```python
from build123d import *

# Parameters (mm, degrees)
F0_W        = 20
F0_H        = 200
F1_DEPTH    = 20
F2_W        = 15
F2_H        = 100
F3_DEPTH    = 20
F6_R        = 7
F7_DEPTH    = 20.001
F8_T1_DEPTH = 20
F9_R        = 20
F11_D       = 6.7564
F11_DEPTH   = 50
F11_TIP     = 2.0298273432


# Not quite as in the source:
# - a fillet or chamfer that OpenCascade refuses, or shapes differently, is made with other operations: its cross-section is extruded or revolved along the edge and cut away or added


with BuildPart() as f1:
    # F0 (on Front) → F1 (new body)
    with BuildSketch(Plane.XZ):
        with Locations((10, 100)):
            Rectangle(F0_W, F0_H)
    extrude(amount=F1_DEPTH)

    # F2 (on face) → F3 (cut)
    with BuildSketch(Plane.YZ.offset(20)):
        with Locations((-12.5, 50)):
            Rectangle(F2_W, F2_H)
    extrude(amount=-F3_DEPTH, mode=Mode.SUBTRACT)

    # F5: sweep along a path in F5_path
    with BuildLine(Plane(origin=(0, -5, 0), x_dir=(0, -1, 0), z_dir=(0, 0, -1))) as f5_path:
        Line((0, 0), (-5, 0))
    # F4 (on face) → F5 (sweep, cut)
    with BuildSketch(Plane(origin=(0, 0, 0), x_dir=(-1, 0, 0), z_dir=(0, 1, 0))):
        with BuildLine():
            Line((0, 0), (0, 10))
            ThreePointArc((0, 10), (-2.9289321881, 2.9289321881), (-10, 0))
            Line((-10, 0), (0, 0))
        make_face()
        with BuildLine():
            ThreePointArc((-10, 0), (-17.0710678277, 2.9289322039), (-20, 10.0000000447))
            Line((-20, 10.0000000447), (-20, 0))
            Line((-20, 0), (-10, 0))
        make_face()
    sweep(path=f5_path.line, mode=Mode.SUBTRACT)

    # F6 (on face) → F7 (cut, through all)
    with BuildSketch(Plane(origin=(0, 0, 0), x_dir=(-1, 0, 0), z_dir=(0, 1, 0))):
        with Locations((-10, 10)):
            Circle(F6_R)
    extrude(amount=-F7_DEPTH, mode=Mode.SUBTRACT)

    # F8: fillet of radius 45 on 1 edges, made by hand

    # F8_s2 → F8_t1 (join)
    with BuildSketch(Plane.YZ):
        with BuildLine():
            ThreePointArc((-5, 66.4589803375), (-8.9208081871, 84.8301534084), (-20, 100))
            Line((-20, 100), (-5, 100))
            Line((-5, 100), (-5, 66.4589803375))
        make_face()
    extrude(amount=F8_T1_DEPTH)

    # F9
    f9_edges = [f1.edges().sort_by_distance(p)[0] for p in [
        (10, -20, 100),
    ]]
    fillet(f9_edges, radius=F9_R)

    # F11
    with Locations(Plane.XY.offset(200)):
        with Locations((10, -10)):
            Hole(F11_D / 2, depth=F11_DEPTH)
            with Locations((0, 0, -(F11_DEPTH + F11_TIP / 2))):  # 118° drill point
                Cone(0, F11_D / 2, F11_TIP, mode=Mode.SUBTRACT)


solid = f1.part
```
Geometry check sheet. Reference: the model listing, model coordinates, mm. A direction names the side the tool comes from. Give positions to 0.01 mm unless a question says otherwise; leave off trailing zeros. Loops run counter-clockwise (first coordinate to the right, second up) from the corner with the lowest first, then second, coordinate; pieces in that order, holes last. Notation, with made-up numbers: M 44.25,19.5 L 52.25,19.5 A28 ccw 52.25,55.5 Z; hole C 59.5,72.5 d3. An arc over 180 degrees is marked long. Answer as CSV lines item,"result".
Item 1: Cross-section at B-B on z = 61.5. Record the cut outline in (x, y), and give its area (3 significant figures).
Values:
outline,"M 0,-5 L 20,-5 L 20,0 L 0,0 Z"
area,"100 mm²"
Item 2: Access from +Z, -Z, +X, -X, +Y, -Y to the whole of each face (thin tool, end or side, straight path). Record for faces 4 (the flat face through (10, 0, 101)), 5 (the flat face through (10, -5, 33)).
Values:
face 4,"+Z, -Z, +X, -X, +Y"
face 5,"-Z, +X, -X, -Y"
Item 3: Material ranges on line 1 (Z direction, x = 10, y = -3.65); line 2 (Y direction, x = 10, z = 184); line 3 (X direction, y = -10, z = 181.5), recorded low to high.
Values:
line 1,"z = 0 to 3, 17 to 200"
line 2,"y = -20 to -13.38, -6.62 to 0"
line 3,"x = 0 to 6.62, 13.38 to 20"
Item 4: Release check for a two-part mould opening along Y. For faces 1 (the cylindrical face through (10.44, -6.65, 174.65)), 2 (the cylindrical face through (9.86, -7.602, 81.539)), 3 (the flat face through (20, -8, 127)) record: pulls with the +Y half, pulls with the -Y half, needs draft (parallel to the pull), parting line crosses it, or undercut.
Values:
face 1,"undercut"
face 2,"pulls with the -Y half"
face 3,"needs draft"
Item 5: Cross-section at A-A on z = 12.5. Record the cut outline in (x, y), and give its area (3 significant figures).
Values:
outline,"M 0,-5 L 3.46,-5 L 3.46,0 L 0,0 Z; M 16.54,-5 L 20,-5 L 20,0 L 16.54,0 Z"
area,"34.6 mm²"
Item 6: Depth check by flat-ended pin: P1, Ø8.5, axis at x = 10, z = 10, coming from the +Y side; P2, Ø6, axis at x = 10.5, z = 34, coming from the -Y side. Enter the tip coordinate at first touch or a pass-through.
Values:
P1,"passes through"
P2,"stops at y = -5"
Item 7: Cross-section at C-C on z = 104.5. Record the cut outline in (x, y).
Values:
outline,"M 0,-19.69 L 20,-19.69 L 20,0 L 0,0 Z"
